from build123d import *

# Parameters (mm, degrees)
SZKIC1_R                    = 9.5
DODANIE_WYCI_GNI_CIE1_DEPTH = 4.5
ZAOKR_GLENIE1_R             = 0.2


with BuildPart() as part:
    # Szkic1 → Dodanie-wyciągnięcie1 (new body, symmetric)
    with BuildSketch(Plane(origin=(0, 0, 0), x_dir=(1, 0, 0), z_dir=(0, 1, 0))):
        Circle(SZKIC1_R)
    extrude(amount=DODANIE_WYCI_GNI_CIE1_DEPTH, both=True)

    # Szkic3 → Wycięcie-obrót1 (revolve, cut)
    with BuildSketch(Plane.XY):
        with BuildLine():
            Line((0, -7.94), (0, 7.94))
            ThreePointArc((0, 7.94), (7.94, 0), (0, -7.94))
        make_face()
    revolve(axis=Axis((0, -7.94, 0), (0, 1, 0)), mode=Mode.SUBTRACT)

    # Zaokrąglenie1
    zaokr_glenie1_edges = [part.edges().sort_by_distance(p)[0] for p in [
        (-9.5, -4.5, 0),
        (-9.5, 4.5, 0),
    ]]
    fillet(zaokr_glenie1_edges, radius=ZAOKR_GLENIE1_R)


solid = part.part
The model under review builds one solid part; all positions refer to its coordinate system, in mm. Give positions to 0.01 mm unless a question says otherwise; leave off trailing zeros. Order: outer loops, then holes, each group sorted by start corner. A loop starts at its lowest first (then second) coordinate and runs counter-clockwise, first axis right, second up. Notation, with made-up numbers: M -35,-4 L 7,-4 A29 ccw 7,28 Z; hole C 13,61 d8. An arc over 180 degrees is marked long. Use one line per item in the form item = value. Start each with the question number.
Item 1: Insertion check: pin 1 Ø4 at (y, z) = (2.5, -7) entering from +X; pin 2 Ø5 at (x, y) = (-5, 1.5) entering from -Z. Each pin has a flat end and moves straight along its axis. Give the tip position at first contact, or say it passes through.
Item 2: We need section D-D on y = -0.5. Give the boundary of the cut face in (x, z).
Item 3: We need section C-C on y = 1. Give the boundary of the cut face in (x, z).
Item 4: To check wall thickness, follow line 1 along X through (y, z) = (4, -6.25); line 2 along Z through (x, y) = (-2, 2.75); line 3 along X through (y, z) = (2.25, -3). State the ranges of each line that lie inside material, in increasing order. Write a range as from..to.
Item 5: We need section B-B on z = 0. Give the boundary of the cut face in (x, y), plus the area to 3 significant figures.
Item 6: We need section A-A on x = 0. Give the boundary of the cut face in (y, z), plus the area to 3 significant figures.
Completed:
q1.pin_1 = 8.08
q1.pin_2 = -9.17
q2.outline = C 0,0 d19; hole C 0,0 d15.85
q3.outline = C 0,0 d19; hole C 0,0 d15.75
q4.line_1 = -7.15..-2.83, 2.83..7.15
q4.line_2 = -9.29..-7.18, 7.18..9.29
q4.line_3 = -9.01..-7, 7..9.01
q5.outline = M -9.5,-4.3 A0.2 ccw -9.3,-4.5 L -6.54,-4.5 A7.94 cw -6.54,4.5 L -9.3,4.5 A0.2 ccw -9.5,4.3 Z; M 6.54,-4.5 L 9.3,-4.5 A0.2 ccw 9.5,-4.3 L 9.5,4.3 A0.2 ccw 9.3,4.5 L 6.54,4.5 A7.94 cw Z
q5.area = 36.1 mm²
q6.outline = M -4.5,-9.3 A0.2 ccw -4.3,-9.5 L 4.3,-9.5 A0.2 ccw 4.5,-9.3 L 4.5,-6.54 A7.94 cw -4.5,-6.54 Z; M -4.5,6.54 A7.94 cw 4.5,6.54 L 4.5,9.3 A0.2 ccw 4.3,9.5 L -4.3,9.5 A0.2 ccw -4.5,9.3 Z
q6.area = 36.1 mm²
